```python
from build123d import *

# Parameters (mm, degrees)
BOSS_EXTRUDE1_DEPTH = 3
SKETCH2_W           = 1.5
SKETCH2_H           = 115.6
CUT_EXTRUDE1_DEPTH  = 4


with BuildPart() as part:
    # Sketch1 → Boss-Extrude1 (new body)
    with BuildSketch(Plane(origin=(0, 0, 0), x_dir=(1, 0, 0), z_dir=(0, 1, 0))):
        Polygon((0, 0), (17.52857143, 0), (17.52857143, -3), (35.05714243, -3), (35.05714243, 0), (52.58571343, 0), (52.58571343, -3), (70.11428443, -3), (70.11428443, 0), (87.64285543, 0), (87.64285543, -3), (105.17142643, -3), (105.17142643, 0), (122.7, 0), (122.7, 115.6), (105.17142643, 115.6), (105.17142643, 118.6), (87.64285543, 118.6), (87.64285543, 115.6), (70.11428443, 115.6), (70.11428443, 118.6), (52.58571343, 118.6), (52.58571343, 115.6), (35.05714243, 115.6), (35.05714243, 118.6), (17.52857143, 118.6), (17.52857143, 115.6), (0, 115.6), align=None)
    extrude(amount=BOSS_EXTRUDE1_DEPTH)

    # Sketch2 → Cut-Extrude1 (cut, through all)
    with BuildSketch(Plane.XZ):
        with Locations((0.75, -57.8)):
            Rectangle(SKETCH2_W, SKETCH2_H)
    extrude(amount=-CUT_EXTRUDE1_DEPTH, mode=Mode.SUBTRACT)


solid = part.part
```
Geometry: final body of the model. Coordinates: model frame, mm. A direction names the side the tool comes from. Coordinates: 2 decimals unless noted, no trailing zeros. Order: outer loops, then holes, each group sorted by start corner. A loop starts at its lowest first (then second) coordinate and runs counter-clockwise, first axis right, second up. Notation, with made-up numbers: (-3.5, 66.25) -> (8.5, 66.25) arc R26 ccw to (8.5, 95.25) -> close; hole circle Ø2 at (27.25, -34). An arc over 180 degrees is marked (long way). Answer in a Markdown table with one row per item.
Item 1: Access query for faces 5 (the flat face through (114, 1, 0)), 6 (the flat face through (44, 1, -115.6)), 7 (the flat face through (17.529, 1, 1)), 8 (the flat face through (10, 1, -115.6)). Directions: +Z, -Z, +X, -X, +Y, -Y. A direction counts if a zero-diameter tool reaches every point of the face in a straight line with its end or side. Return the directions, or none.
Return value:
| item | result |
|---|---|
| face 5 | +Z, +X, +Y, -Y |
| face 6 | -Z, +Y, -Y |
| face 7 | +Z, -X, +Y, -Y |
| face 8 | -Z, -X, +Y, -Y |
Item 2: Draft query along X for faces 1 (the flat face through (122.7, 1, -57)), 2 (the flat face through (1.5, 1, -59)), 3 (the flat face through (26, 1, 3)), 4 (the flat face through (35.057, 1, 2)). Return one class per face: released by +X, released by -X, zero draft, split by the parting line, or undercut.
Return value:
| item | result |
|---|---|
| face 1 | released by +X |
| face 2 | released by -X |
| face 3 | zero draft |
| face 4 | undercut |
Item 3: Section B-B on x = 44.5. Output: boundary loops of the cut face in (y, z).
Return value:
| item | result |
|---|---|
| outline | (0, -115.6) -> (3, -115.6) -> (3, 0) -> (0, 0) -> close |
Item 4: Contact query for flat-ended pins moving along their axis: P1, Ø1.5, axis at y = 1, z = -117, coming from the -X side; P2, Ø0.9, axis at y = 1.5, z = -116.5, coming from the +X side; P3, Ø0.9, axis at x = 116, y = 1, coming from the -Z side. Output: stop coordinate, or through.
Return value:
| item | result |
|---|---|
| P1 | stops at x = 17.53 |
| P2 | stops at x = 105.17 |
| P3 | stops at z = -115.6 |
Item 5: Section A-A on y = 1.65. Output: boundary loops of the cut face in (x, z).
Return value:
| item | result |
|---|---|
| outline | (1.5, -115.6) -> (17.53, -115.6) -> (17.53, -118.6) -> (35.06, -118.6) -> (35.06, -115.6) -> (52.59, -115.6) -> (52.59, -118.6) -> (70.11, -118.6) -> (70.11, -115.6) -> (87.64, -115.6) -> (87.64, -118.6) -> (105.17, -118.6) -> (105.17, -115.6) -> (122.7, -115.6) -> (122.7, 0) -> (105.17, 0) -> (105.17, 3) -> (87.64, 3) -> (87.64, 0) -> (70.11, 0) -> (70.11, 3) -> (52.59, 3) -> (52.59, 0) -> (35.06, 0) -> (35.06, 3) -> (17.53, 3) -> (17.53, 0) -> (1.5, 0) -> close |
Item 6: Ray query, L1, parallel to Z at x = 114, y = 1.9. Return the intervals inside material, ascending.
Return value:
| item | result |
|---|---|
| L1 | z = -115.6 to 0 |
